from build123d import *

# Parameters (mm, degrees)
SKETCH1_W                 = 50.8
SKETCH1_H                 = 38.1
BOSS_EXTRUDE1_DEPTH       = 6.35
SKETCH3_R                 = 1.8288
CUT_EXTRUDE1_DEPTH        = 6.35
F_6_32_TAPPED_HOLE1_D     = 2.7051
F_6_32_TAPPED_HOLE1_DEPTH = 11.88730597
F_6_32_TAPPED_HOLE1_TIP   = 0.81269403
SKETCH12_R                = 3.175
CUT_EXTRUDE3_DEPTH        = 6.35


with BuildPart() as part:
    # Sketch1 → Boss-Extrude1 (new body)
    with BuildSketch(Plane(origin=(0, 0, 0), x_dir=(0, 0, -1), z_dir=(1, 0, 0))):
        with Locations((-25.4, 19.05)):
            Rectangle(SKETCH1_W, SKETCH1_H)
    extrude(amount=BOSS_EXTRUDE1_DEPTH)

    # Sketch3 → Cut-Extrude1 (cut)
    with BuildSketch(Plane(origin=(6.35, 0, 0), x_dir=(0, 0, -1), z_dir=(1, 0, 0))):
        with Locations((-44.45, 3.175)):
            Circle(SKETCH3_R)
        with Locations((-25.4, 3.175)):
            Circle(SKETCH3_R)
        with Locations((-6.35, 3.175)):
            Circle(SKETCH3_R)
    extrude(amount=-CUT_EXTRUDE1_DEPTH, mode=Mode.SUBTRACT)

    # #6-32 Tapped Hole1
    with Locations(Plane(origin=(0, 38.1, 0), x_dir=(1, 0, 0), z_dir=(0, 1, 0))):
        with Locations((3.175, -6.35), (3.175, -25.4), (3.175, -44.45)):
            Hole(F_6_32_TAPPED_HOLE1_D / 2, depth=F_6_32_TAPPED_HOLE1_DEPTH)
            with Locations((0, 0, -(F_6_32_TAPPED_HOLE1_DEPTH + F_6_32_TAPPED_HOLE1_TIP / 2))):  # 118° drill point
                Cone(0, F_6_32_TAPPED_HOLE1_D / 2, F_6_32_TAPPED_HOLE1_TIP, mode=Mode.SUBTRACT)

    # Sketch12 → Cut-Extrude3 (cut)
    with BuildSketch(Plane(origin=(6.35, 0, 0), x_dir=(0, 0, -1), z_dir=(1, 0, 0))):
        with Locations((-25.4, 17.653)):
            Circle(SKETCH12_R)
    extrude(amount=-CUT_EXTRUDE3_DEPTH, mode=Mode.SUBTRACT)


solid = part.part
Input: part model. Units: mm. Frame: model coordinates. A direction names the side the tool comes from. Coordinates: 2 decimals unless noted, no trailing zeros. Loops run counter-clockwise (first coordinate to the right, second up) from the corner with the lowest first, then second, coordinate; pieces in that order, holes last.
(1) Section A-A on y = 27. Return the cut outline in (x, z) (3 decimals).
(2) Material intervals for probe 1 along Z at (x, y) = (1.25, 3); probe 2 along Y at (x, z) = (1.5, 25.4); probe 3 along Y at (x, z) = (3, 24.5), sorted ascending.
(3) Set-up query: faces 1 (the face through (3.47, 32.07, 26.72)), 2 (the face through (3, 19, 0)). Return all of +Z, -Z, +X, -X, +Y, -Y with unobstructed straight access to the full face (end or side cutting, diameter ignored); none if empty.
(4) First-contact query: pin 1 Ø2.5 at (x, z) = (3.175, 6.35) entering from +Y; pin 2 Ø6 at (y, z) = (3.175, 44.45) entering from +X; pin 3 Ø1.6 at (x, z) = (3.175, 44.45) entering from +Y. Flat tips, straight axial feed; report the tip coordinate or a pass-through.
(5) Pull-direction query (X, two-part tool) for faces 3 (the face through (6.35, 24, 26)), 4 (the face through (3.219, 3.255, 46.277)), 5 (the face through (3.28, 25.54, 44.66)); classes: released by +X, released by -X, zero draft, split by the parting line, or undercut.
Data:
1. outline: (0, 0) - (6.35, 0) - (6.35, 50.8) - (0, 50.8) - close; hole circle Ø2.705 at (3.175, 6.35); hole circle Ø2.705 at (3.175, 25.4); hole circle Ø2.705 at (3.175, 44.45)
2. probe 1: z = 0 to 4.53, 8.17 to 23.58, 27.22 to 42.63, 46.27 to 50.8
2. probe 2: y = 0 to 1.35, 5 to 14.48, 20.83 to 38.1
2. probe 3: y = 0 to 1.58, 4.77 to 14.61, 20.7 to 25.95
3. face 1: +Y
3. face 2: -Z, +X, -X, +Y, -Y
4. pin 1: stops at y = 26.15
4. pin 2: stops at x = 6.35
4. pin 3: stops at y = 25.88
5. face 3: released by +X
5. face 4: zero draft
5. face 5: undercut
